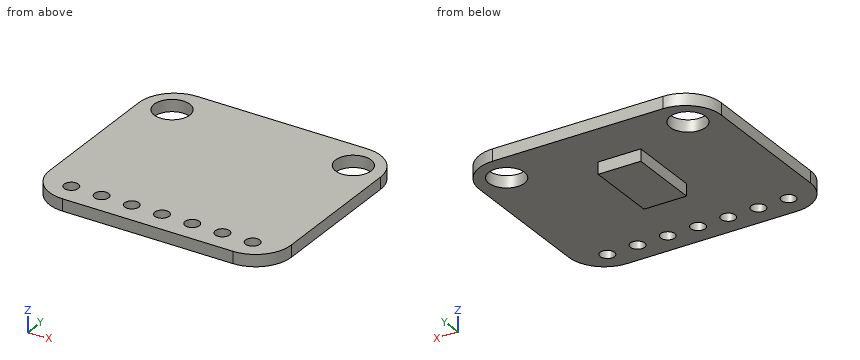
from build123d import *

# Parameters (mm, degrees)
SKETCH_1_W           = 20.32
SKETCH_1_H           = 17.78
SKETCH_1_R           = 1.5
SKETCH_1_R_2         = 0.6
EXTRUDE_1_DEPTH      = 1
FILLET_2_R           = 3
FILLET_3_R           = 3
FILLET_4_R           = 3
FILLET_5_R           = 3
EXTRUDE_2_DEPTH      = 1
EXTRUDE_2_DEPTH_BACK = 1
SKETCH_2_W           = 3.580076994
SKETCH_2_H           = 6.056150923


with BuildPart() as part:
    # 草图1 → 凸台-拉伸1 (new body)
    with BuildSketch(Plane.XY):
        Rectangle(SKETCH_1_W, SKETCH_1_H)
        with Locations((-7.62, 6.303875277)):
            Circle(SKETCH_1_R, mode=Mode.SUBTRACT)
        with Locations((7.62, 6.303875277)):
            Circle(SKETCH_1_R, mode=Mode.SUBTRACT)
        with Locations((-7.62, -7.003605695)):
            Circle(SKETCH_1_R_2, mode=Mode.SUBTRACT)
        with Locations((-5.08, -7.003605695)):
            Circle(SKETCH_1_R_2, mode=Mode.SUBTRACT)
        with Locations((-2.54, -7.003605695)):
            Circle(SKETCH_1_R_2, mode=Mode.SUBTRACT)
        with Locations((0, -7.003605695)):
            Circle(SKETCH_1_R_2, mode=Mode.SUBTRACT)
        with Locations((2.54, -7.003605695)):
            Circle(SKETCH_1_R_2, mode=Mode.SUBTRACT)
        with Locations((5.08, -7.003605695)):
            Circle(SKETCH_1_R_2, mode=Mode.SUBTRACT)
        with Locations((7.62, -7.003605695)):
            Circle(SKETCH_1_R_2, mode=Mode.SUBTRACT)
    extrude(amount=EXTRUDE_1_DEPTH)

    # 圆角2
    fillet_2_edges = [part.edges().sort_by_distance(p)[0] for p in [
        (10.16, 8.89, 0.5),
    ]]
    fillet(fillet_2_edges, radius=FILLET_2_R)

    # 圆角3
    fillet_3_edges = [part.edges().sort_by_distance(p)[0] for p in [
        (-10.16, 8.89, 0.5),
    ]]
    fillet(fillet_3_edges, radius=FILLET_3_R)

    # 圆角4
    fillet_4_edges = [part.edges().sort_by_distance(p)[0] for p in [
        (-10.16, -8.89, 0.5),
    ]]
    fillet(fillet_4_edges, radius=FILLET_4_R)

    # 圆角5
    fillet_5_edges = [part.edges().sort_by_distance(p)[0] for p in [
        (10.16, -8.89, 0.5),
    ]]
    fillet(fillet_5_edges, radius=FILLET_5_R)

    # 草图2 → 凸台-拉伸2 (add, two sides: drawn at the far end of the back side and taken through both)
    with BuildSketch(Plane.XY.offset(-EXTRUDE_2_DEPTH_BACK)):
        with Locations((-0.887963615, 1.742289852)):
            Rectangle(SKETCH_2_W, SKETCH_2_H)
    extrude(amount=EXTRUDE_2_DEPTH + EXTRUDE_2_DEPTH_BACK)


solid = part.part
Source: CAD feature listing. Evaluate the final solid. Frame: model axes, mm. Give positions to 0.01 mm unless a question says otherwise; leave off trailing zeros. Write each loop counter-clockwise with the first axis right and the second up, starting at its lowest first coordinate (ties: lowest second). Pieces come first, ordered by that corner, then holes. Notation, with made-up numbers: (-17.75, 74) -> (20.25, 74) arc R12 cw to (20.25, 88) -> close; hole circle Ø9 at (3.5, -15). An arc over 180 degrees is marked (long way). Write item = value, one per line.
Q1. Line query: line 1 (Y direction, x = 0, z = 0.8); line 2 (Y direction, x = -7.62, z = 0.5); line 3 (X direction, y = 7, z = 0.5). Output: solid intervals per line, ascending. Write a range as from..to.
Here are the results:
line_1 = -8.89..-7.6, -6.4..8.89
line_2 = -8.85..-7.6, -6.4..4.8, 7.8..8.85
line_3 = -9.95..-8.95, -6.29..6.29, 8.95..9.95
Q2. Cut plane C-C on x = -7.62. Return loops of the section in (y, z), then the cut area to 3 significant figures.
Here are the results:
outline = (-8.85, 0) -> (-7.6, 0) -> (-7.6, 1) -> (-8.85, 1) -> close; (-6.4, 0) -> (4.8, 0) -> (4.8, 1) -> (-6.4, 1) -> close; (7.8, 0) -> (8.85, 0) -> (8.85, 1) -> (7.8, 1) -> close
area = 13.5 mm²
Q3. Cut plane B-B on y = 2.5. Return loops of the section in (x, z), then the cut area to 3 significant figures.
Here are the results:
outline = (-10.16, 0) -> (-2.68, 0) -> (-2.68, -1) -> (0.9, -1) -> (0.9, 0) -> (10.16, 0) -> (10.16, 1) -> (-10.16, 1) -> close
area = 23.9 mm²
Q4. First-contact query: pin 1 (0.5 mm diameter, centred on y = 2.5, z = -0.5, fed in from +X); pin 2 (1 mm diameter, centred on x = -5, y = -5, fed in from -Z); pin 3 (0.5 mm diameter, centred on x = -1.5, z = -0.5, fed in from -Y). Flat tips, straight axial feed; report the tip coordinate or a pass-through.
Here are the results:
pin_1 = 0.9
pin_2 = 0
pin_3 = -1.29
Q5. Cut plane D-D on z = 0.4. State how many separate pieces and enclosed holes the cut face has, then the cut area to 3 significant figures.
Here are the results:
separate_pieces = 1
enclosed_holes = 9
area = 332 mm²
Q6. Cut plane A-A on x = 5.08. Return loops of the section in (y, z), then the cut area to 3 significant figures.
Here are the results:
outline = (-8.89, 0) -> (-7.6, 0) -> (-7.6, 1) -> (-8.89, 1) -> close; (-6.4, 0) -> (8.89, 0) -> (8.89, 1) -> (-6.4, 1) -> close
area = 16.6 mm²
